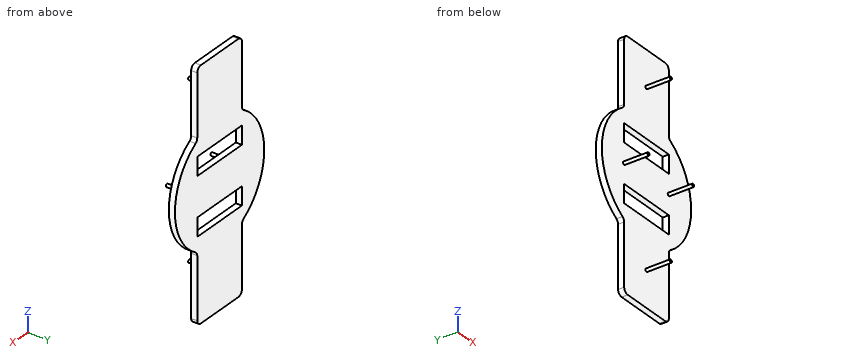
from build123d import *

# Parameters (mm, degrees)
F1_DEPTH = 6.35
F2_R     = 5.08
F3_W     = 63.5
F3_H     = 19.05
F4_DEPTH = 25.4
F5_R     = 1.5875
F6_DEPTH = 25.4


with BuildPart() as f1:
    # F0 (on Front) → F1 (new body)
    with BuildSketch(Plane.XZ):
        with BuildLine():
            ThreePointArc((31.75, -54.9926131403), (54.9926131403, -31.75), (63.5, 0))
            ThreePointArc((63.5, 0), (54.9926131403, 31.75), (31.75, 54.9926131403))
            Line((31.75, 54.9926131403), (31.75, -54.9926131403))
        make_face()
        with BuildLine():
            Line((31.75, -54.9926131403), (31.75, 54.9926131403))
            ThreePointArc((31.75, 54.9926131403), (0, 63.5), (-31.75, 54.9926131403))
            Line((-31.75, 54.9926131403), (-31.75, -54.9926131403))
            ThreePointArc((-31.75, -54.9926131403), (0, -63.5), (31.75, -54.9926131403))
        make_face()
        with BuildLine():
            ThreePointArc((-31.75, 54.9926131403), (0, 63.5), (31.75, 54.9926131403))
            Line((31.75, 54.9926131403), (31.75, 127))
            Line((31.75, 127), (-31.75, 127))
            Line((-31.75, 127), (-31.75, 54.9926131403))
        make_face()
        with BuildLine():
            Line((31.75, -127), (31.75, -54.9926131403))
            ThreePointArc((31.75, -54.9926131403), (0, -63.5), (-31.75, -54.9926131403))
            Line((-31.75, -54.9926131403), (-31.75, -127))
            Line((-31.75, -127), (31.75, -127))
        make_face()
        with BuildLine():
            Line((-31.75, -54.9926131403), (-31.75, 54.9926131403))
            ThreePointArc((-31.75, 54.9926131403), (-63.5, 0), (-31.75, -54.9926131403))
        make_face()
    extrude(amount=F1_DEPTH)

    # F2
    f2_edges = [f1.edges().sort_by_distance(p)[0] for p in [
        (31.75, -3.175, 54.992613),
        (-31.75, -3.175, 54.992613),
        (-31.75, -3.175, -54.992613),
        (31.75, -3.175, -54.992613),
        (31.75, -3.175, 127),
        (-31.75, -3.175, 127),
        (31.75, -3.175, -127),
        (-31.75, -3.175, -127),
    ]]
    fillet(f2_edges, radius=F2_R)

    # F3 (on face) → F4 (cut)
    with BuildSketch(Plane.XZ.offset(6.35)):
        with Locations((0, 29.8867885709)):
            Rectangle(F3_W, F3_H)
        with Locations((0, -29.8867885709)):
            Rectangle(F3_W, F3_H)
    extrude(amount=-F4_DEPTH, mode=Mode.SUBTRACT)

    # F5 (on face) → F6 (join)
    with BuildSketch(Plane.XZ.offset(6.35)):
        with Locations((-31.75, 0)):
            Circle(F5_R)
        with Locations((31.75, 0)):
            Circle(F5_R)
        with Locations((0, -89.8856266138)):
            Circle(F5_R)
        with Locations((0, 89.8856266138)):
            Circle(F5_R)
    extrude(amount=F6_DEPTH)


solid = f1.part
Could you check a few things on this model? Use its own coordinates, in mm. Coordinates: 2 decimals unless noted, no trailing zeros. Order: outer loops, then holes, each group sorted by start corner. A loop starts at its lowest first (then second) coordinate and runs counter-clockwise, first axis right, second up.
Q1. Suppose I cut it at D-D on x = -46. Please give me the cut outline in (y, z) (3 decimals), and give its area (3 significant figures).
Q2. Please list where these lines run through material, in increasing order: L1, parallel to Z at x = -7, y = -0.5; L2, parallel to Y at x = -55, z = -5; L3, parallel to Z at x = 31.5, y = -25.5.
Q3. Suppose I cut it at B-B on z = -62. Please give me the cut outline in (x, y).
Q4. Will these pins go through, and if not, where does the flat tip stop? pin 1 (5 mm diameter, centred on y = -4, z = 32.5, fed in from -X); pin 2 (1.9 mm diameter, centred on y = -2, z = -27, fed in from +X); pin 3 (5 mm diameter, centred on y = -2, z = -104.5, fed in from +X).
Q5. Suppose I cut it at C-C on y = -27.5. Give the number of separate pieces and of enclosed holes in the cut face, and give its area (3 significant figures).
Q6. Suppose I cut it at A-A on x = -21. Please give me the cut outline in (y, z), and give its area (3 significant figures).
Answer:
1. outline: (-6.35, -43.775) - (0, -43.775) - (0, 43.775) - (-6.35, 43.775) - close
1. area: 556 mm2
2. L1: z = -127 to -39.41, -20.36 to 20.36, 39.41 to 127
2. L2: y = -6.35 to 0
2. L3: z = -1.57 to 1.57
3. outline: (-31.75, -6.35) - (31.75, -6.35) - (31.75, 0) - (-31.75, 0) - close
4. pin 1: stops at x = -55.97
4. pin 2: stops at x = 57.91
4. pin 3: stops at x = 31.75
5. separate pieces: 4
5. enclosed holes: 0
5. area: 31.7 mm2
6. outline: (-6.35, -127) - (0, -127) - (0, -39.41) - (-6.35, -39.41) - close; (-6.35, -20.36) - (0, -20.36) - (0, 20.36) - (-6.35, 20.36) - close; (-6.35, 39.41) - (0, 39.41) - (0, 127) - (-6.35, 127) - close
6. area: 1,370 mm2
